Part model, mm, in its own coordinate system. A direction names the side the tool comes from. Round coordinates to 2 decimals unless told otherwise and drop trailing zeros. Write each loop counter-clockwise with the first axis right and the second up, starting at its lowest first coordinate (ties: lowest second). Pieces come first, ordered by that corner, then holes.
1) Saw through at B-B on z = -10. Write the cut outline in (x, y), and give its area (3 significant figures).
2) Saw through at D-D on x = 0. Write the cut outline in (y, z), and give its area (3 significant figures).
3) Flat gauge pins, fed straight in: pin 1 (3.5 mm diameter, centred on x = -8.5, y = 8.5, fed in from -Z); pin 2 (1.5 mm diameter, centred on x = 0.5, y = -8, fed in from -Z); pin 3 (2.5 mm diameter, centred on x = -7.5, z = -10, fed in from -Y); pin 4 (5 mm diameter, centred on x = -4.5, z = -8.5, fed in from +Y). Where does each tip first touch, or does it go through?
4) Pull direction X, two halves, no side cores. Call faces 4 (the cylindrical face through (-8.85, -10.06, 1.48)), 5 (the flat face through (-3, -13, -20)), 6 (the cylindrical face through (11.9, -13.02, -19.43)): +X half, -X half, draft (parallel to the pull), parting line (faces both ways), or undercut.
5) Which spindle directions (+Z, -Z, +X, -X, +Y, -Y) get a long thin tool onto all of the face, cutting with end or side? Do faces 1 (the flat face through (5, -11, -1)), 2 (the cylindrical face through (-16.93, -13.02, -19.4)), 3 (the flat face through (-12.5, -1, 1)). Say none if no direction does.
6) Saw through at C-C on x = 8.5. Write the cut outline in (y, z), and give its area (3 significant figures).
7) Saw through at A-A on y = 8.5. Write the cut outline in (x, z).
8) Drill centre lines: L1, parallel to Y at x = 8.5, z = 2.2; L2, parallel to Z at x = -7.5, y = -12.8; L3, parallel to X at y = 0.25, z = 1.5. Where is each one in solid material? Low to high.
```python
from build123d import *

# Parameters (mm, degrees)
SKETCH_R     = 7.65
SKETCH_R_2   = 1.6
PAD_DEPTH    = 3
SKETCH001_W  = 30
SKETCH001_H  = 3
PAD001_DEPTH = 20
SKETCH002_R  = 1.5
POCKET_DEPTH = 27.001
PAD002_DEPTH = 5
FILLET_R     = 2
FILLET001_R  = 2
FILLET002_R  = 2


with BuildPart() as part:
    # Sketch → Pad (new body)
    with BuildSketch(Plane.XY):
        Polygon((-12.5, -11.5), (-12.5, 12.5), (12.5, 12.5), (12.5, -14.5), (-17.5, -14.5), (-17.5, -11.5), align=None)
        Circle(SKETCH_R, mode=Mode.SUBTRACT)
        with Locations((-8.5, 8.5)):
            Circle(SKETCH_R_2, mode=Mode.SUBTRACT)
        with Locations((8.5, 8.5)):
            Circle(SKETCH_R_2, mode=Mode.SUBTRACT)
        with Locations((8.5, -8.5)):
            Circle(SKETCH_R_2, mode=Mode.SUBTRACT)
        with Locations((-8.5, -8.5)):
            Circle(SKETCH_R_2, mode=Mode.SUBTRACT)
    extrude(amount=PAD_DEPTH)

    # Sketch001 (on Face12 of Pad) → Pad001 (join)
    with BuildSketch(Plane(origin=(0, 0, 0), x_dir=(1, 0, 0), z_dir=(0, 0, -1))):
        with Locations((-2.5, 13)):
            Rectangle(SKETCH001_W, SKETCH001_H)
    extrude(amount=PAD001_DEPTH)

    # Sketch002 (on Face18 of Pad001) → Pocket (cut, through all)
    with BuildSketch(Plane.XZ.offset(14.5)):
        with Locations((-12.5, -10)):
            Circle(SKETCH002_R)
        with Locations((-7.5, -10)):
            Circle(SKETCH002_R)
    extrude(amount=-POCKET_DEPTH, mode=Mode.SUBTRACT)

    # Sketch003 (on Face16 of Pocket) → Pad002 (join, symmetric)
    with BuildSketch(Plane.YZ):
        Polygon((-11.5, 0), (-8.5, 0), (-11.5, -3), align=None)
    extrude(amount=PAD002_DEPTH, both=True)

    # Fillet
    fillet_edges = [part.edges().sort_by_distance(p)[0] for p in [
        (-17.5, -13, 3),
    ]]
    fillet(fillet_edges, radius=FILLET_R)

    # Fillet001
    fillet001_edges = [part.edges().sort_by_distance(p)[0] for p in [
        (12.5, -13, -20),
        (-17.5, -13, -20),
    ]]
    fillet(fillet001_edges, radius=FILLET001_R)

    # Fillet002
    fillet002_edges = [part.edges().sort_by_distance(p)[0] for p in [
        (12.5, 12.5, 1.5),
        (-12.5, 12.5, 1.5),
    ]]
    fillet(fillet002_edges, radius=FILLET002_R)


solid = part.part
```
Completed:
1. outline: (-17.5, -14.5) - (-14, -14.5) - (-14, -11.5) - (-17.5, -11.5) - close; (-11, -14.5) - (-9, -14.5) - (-9, -11.5) - (-11, -11.5) - close; (-6, -14.5) - (12.5, -14.5) - (12.5, -11.5) - (-6, -11.5) - close
1. area: 72.0 mm2
2. outline: (-14.5, -20) - (-11.5, -20) - (-11.5, -3) - (-8.5, 0) - (-7.65, 0) - (-7.65, 3) - (-14.5, 3) - close; (7.65, 0) - (12.5, 0) - (12.5, 3) - (7.65, 3) - close
2. area: 99.6 mm2
3. pin 1: stops at z = 0
3. pin 2: stops at z = -0.25
3. pin 3: passes through
3. pin 4: stops at y = -11.5
4. face 4: undercut
4. face 5: draft
4. face 6: +X half
5. face 1: -Z, +X, +Y
5. face 2: -Z, -X, +Y, -Y
5. face 3: +Z, -Z, -X, +Y
6. outline: (-14.5, -20) - (-11.5, -20) - (-11.5, 0) - (-10.1, 0) - (-10.1, 3) - (-14.5, 3) - close; (-6.9, 0) - (6.9, 0) - (6.9, 3) - (-6.9, 3) - close; (10.1, 0) - (12.5, 0) - (12.5, 3) - (10.1, 3) - close
6. area: 122 mm2
7. outline: (-12.5, 0) - (-10.1, 0) - (-10.1, 3) - (-12.5, 3) - close; (-6.9, 0) - (6.9, 0) - (6.9, 3) - (-6.9, 3) - close; (10.1, 0) - (12.5, 0) - (12.5, 3) - (10.1, 3) - close
8. L1: y = -14.5 to -10.1, -6.9 to 6.9, 10.1 to 12.5
8. L2: z = -20 to -11.5, -8.5 to 3
8. L3: x = -12.5 to -7.65, 7.65 to 12.5
